from build123d import *

# Parameters (mm, degrees)
FILLET1_R = 0.6


with BuildPart() as part:
    # Sketch1 → Revolve1 (revolve)
    with BuildSketch(Plane.XY):
        with BuildLine():
            ThreePointArc((2.5, 5.4), (0, 6.602501564), (-2.5, 5.4))
            Line((-2.5, 5.4), (-6, 5.4))
            Line((-6, 5.4), (-6, 9))
            Line((-6, 9), (6, 9))
            Line((6, 9), (6, 5.4))
            Line((6, 5.4), (2.5, 5.4))
        make_face()
    revolve(axis=Axis((6, -12, 0), (-1, 0, 0)))

    # Fillet1
    fillet1_edges = [part.edges().sort_by_distance(p)[0] for p in [
        (-6, -33, 0),
        (6, -33, 0),
    ]]
    fillet(fillet1_edges, radius=FILLET1_R)


solid = part.part
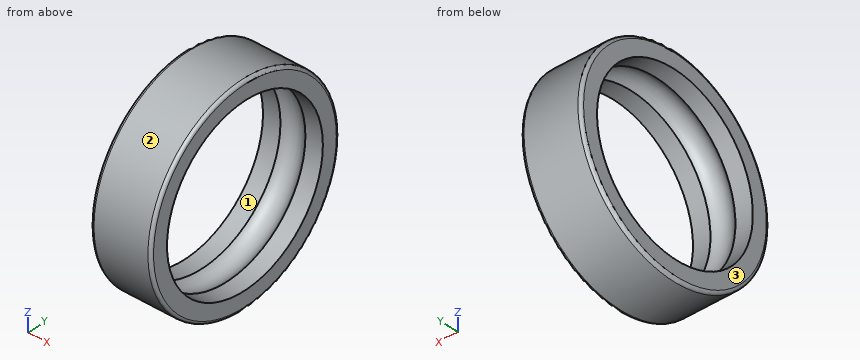
Verification items for the finished model (mm, model axes). Face numbers are marked on the shaded views. Give positions to 0.01 mm unless a question says otherwise; leave off trailing zeros. Write each loop counter-clockwise with the first axis right and the second up, starting at its lowest first coordinate (ties: lowest second). Pieces come first, ordered by that corner, then holes. Notation, with made-up numbers: (40, 27) -> (56, 27) arc R26 cw to (56, 65) -> close; hole circle Ø7 at (-37, 57). An arc over 180 degrees is marked (long way). Use CSV: the item, a comma, the result in double quotes.
(1) Go/stop test with flat-tipped pins: pin 1 (6 mm diameter, centred on x = -1, z = -3.5, fed in from +Y); pin 2 (4 mm diameter, centred on x = -1, z = 14, fed in from +Y); pin 3 (1 mm diameter, centred on x = -2.5, y = -22, fed in from -Z). Record where each tip stops, or that it passes through.
Derived:
pin 1,"stops at y = 8.99"
pin 2,"stops at y = 5.23"
pin 3,"stops at z = -18.73"
(2) Sectioned sample at D-D (x = 3.5). Record the cut outline in (y, z), plus the area to 3 significant figures.
Derived:
outline,"circle Ø42 at (-12, 0); hole circle Ø34.8 at (-12, 0)"
area,"434 mm^2"
(3) Sectioned sample at A-A (y = -12). Record the cut outline in (x, z).
Derived:
outline,"(-6, -20.4) arc R0.6 ccw to (-5.4, -21) -> (5.4, -21) arc R0.6 ccw to (6, -20.4) -> (6, -17.4) -> (2.5, -17.4) arc R3.2 cw to (-2.5, -17.4) -> (-6, -17.4) -> close; (-6, 17.4) -> (-2.5, 17.4) arc R3.2 cw to (2.5, 17.4) -> (6, 17.4) -> (6, 20.4) arc R0.6 ccw to (5.4, 21) -> (-5.4, 21) arc R0.6 ccw to (-6, 20.4) -> close"
(4) Material ranges on L1, parallel to Y at x = -4.4, z = 0; L2, parallel to Z at x = -4.15, y = -12; L3, parallel to Z at x = -5, y = -5, recorded low to high.
Derived:
L1,"y = -33 to -29.4, 5.4 to 9"
L2,"z = -21 to -17.4, 17.4 to 21"
L3,"z = -19.8 to -15.93, 15.93 to 19.8"
(5) Sectioned sample at B-B (z = 0). Record the cut outline in (x, y).
Derived:
outline,"(-6, -32.4) arc R0.6 ccw to (-5.4, -33) -> (5.4, -33) arc R0.6 ccw to (6, -32.4) -> (6, -29.4) -> (2.5, -29.4) arc R3.2 cw to (-2.5, -29.4) -> (-6, -29.4) -> close; (-6, 5.4) -> (-2.5, 5.4) arc R3.2 cw to (2.5, 5.4) -> (6, 5.4) -> (6, 8.4) arc R0.6 ccw to (5.4, 9) -> (-5.4, 9) arc R0.6 ccw to (-6, 8.4) -> close"
(6) Release check for a two-part mould opening along Z. For the marked faces 1, 2 and 3 record: +Z half, -Z half, draft (parallel to the pull), parting line (faces both ways), or undercut.
Derived:
face 1,"undercut"
face 2,"parting line"
face 3,"draft"
(7) Sectioned sample at C-C (x = 0). Record the cut outline in (y, z) (1 decimal).
Derived:
outline,"circle Ø42 at (-12, 0); hole circle Ø37.2 at (-12, 0)"
